Could you check a few things on this drawing? It's one solid part, dimensions in mm from its lowest x, y, z. Give positions to 0.01 mm unless a question says otherwise; leave off trailing zeros. Loops run counter-clockwise (first coordinate to the right, second up) from the corner with the lowest first, then second, coordinate; pieces in that order, holes last.
1. Imagine slicing it at C-C (x = 2.25). List the corners of the cut face in (y, z) for me, plus the area to 3 significant figures.
2. I need wall thicknesses on line 1 along Y through (x, z) = (12.75, 50); line 2 along Z through (x, y) = (17, 50); line 3 along Y through (x, z) = (6.75, 150). Which ranges of each line are inside material? Lowest first, please.
3. Imagine slicing it at A-A (x = 16.25). List the corners of the cut face in (y, z) for me.
4. For P1, Ø11, axis at y = 125, z = 125, coming from the -X side; P2, Ø9.5, axis at y = 50, z = 50, coming from the +X side; P3, Ø7, axis at y = 125, z = 50, coming from the +X side; P4, Ø9.5, axis at y = 150, z = 150, coming from the -X side, each with a flat end and sliding along its axis, tell me the tip position at first contact or that it passes through.
5. Imagine slicing it at B-B (y = 77). List the corners of the cut face in (x, z) for me, plus the area to 3 significant figures.
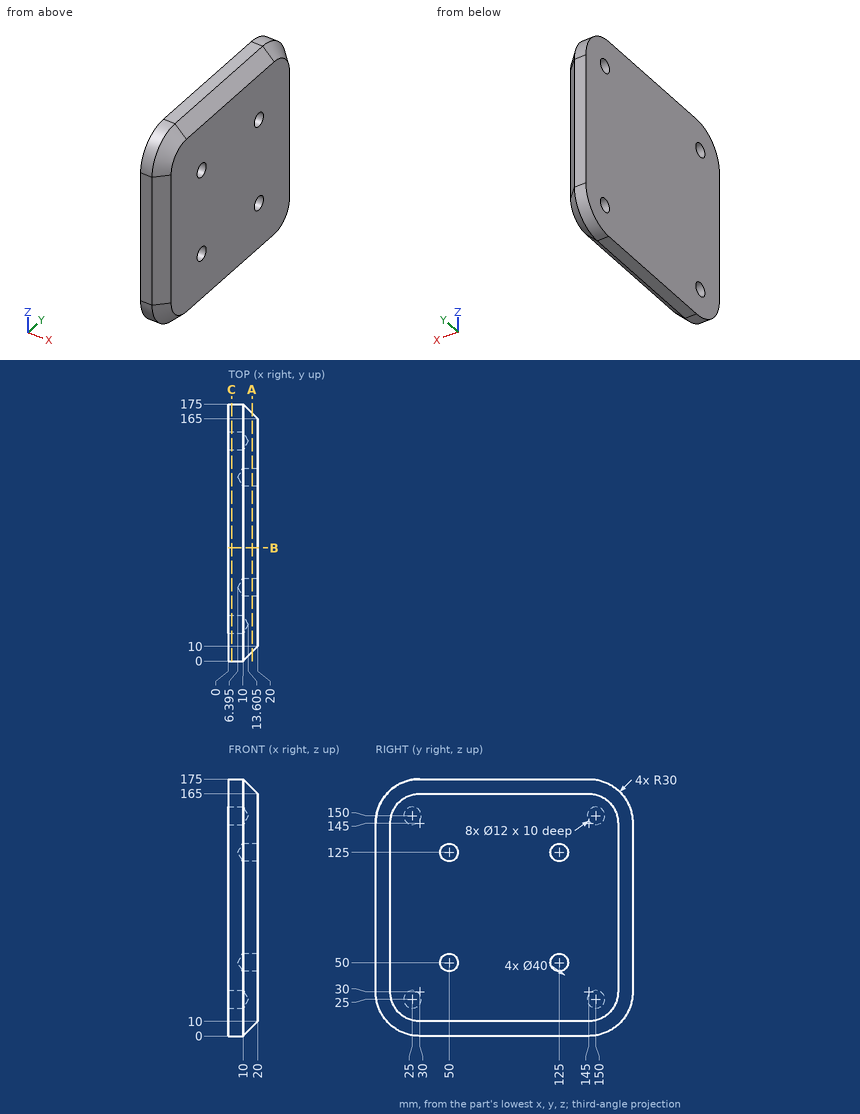
Derived:
1. outline: (0, 30) arc R30 ccw to (30, 0) - (145, 0) arc R30 ccw to (175, 30) - (175, 145) arc R30 ccw to (145, 175) - (30, 175) arc R30 ccw to (0, 145) - close; hole circle Ø12 at (25, 25); hole circle Ø12 at (25, 150); hole circle Ø12 at (150, 25); hole circle Ø12 at (150, 150)
1. area: 29,400 mm2
2. line 1: y = 2.75 to 44, 56 to 119, 131 to 172.25
2. line 2: z = 7 to 44, 56 to 119, 131 to 168
2. line 3: y = 0.42 to 19, 31 to 144, 156 to 174.58
3. outline: (6.25, 30) arc R23.75 ccw to (30, 6.25) - (145, 6.25) arc R23.75 ccw to (168.75, 30) - (168.75, 145) arc R23.75 ccw to (145, 168.75) - (30, 168.75) arc R23.75 ccw to (6.25, 145) - close; hole circle Ø12 at (50, 50); hole circle Ø12 at (50, 125); hole circle Ø12 at (125, 50); hole circle Ø12 at (125, 125)
4. P1: stops at x = 0
4. P2: stops at x = 9.25
4. P3: stops at x = 8.5
4. P4: stops at x = 10.75
5. outline: (0, 0) - (10, 0) - (20, 10) - (20, 165) - (10, 175) - (0, 175) - close
5. area: 3,400 mm2
